Can you work these out from the drawing? Everything is in mm from the part's minimum corner. A direction names the side the tool comes from. Round coordinates to 2 decimals unless told otherwise and drop trailing zeros. Write each loop counter-clockwise with the first axis right and the second up, starting at its lowest first coordinate (ties: lowest second). Pieces come first, ordered by that corner, then holes. Notation, with made-up numbers: (81, -32.5) - (114, -32.5) arc R24 ccw to (114, -15.5) - close; hole circle Ø4 at (79, -20.5). An arc over 180 degrees is marked (long way). One line per item, written item: value. Start each with the question number.
Item 1: Thinking about a two-plate mould opening in Y: for the marked faces 1, 2 and 3, which applies, released by +Y, released by -Y, zero draft, split by the parting line, or undercut?
Item 2: For the marked faces 4, 5 and 6, which set-ups out of +Z, -Z, +X, -X, +Y, -Y let a thin tool reach every point of the face, with its end or its side?
Item 3: Imagine slicing it at B-B, the plane z = 1.5. Please give me the cut outline in (x, y), then the cut area to 3 significant figures.
Item 4: If I drill on line 1 (Z direction, x = 2.5, y = 20) (3 decimals); line 2 (Z direction, x = 2.5, y = 43) (3 decimals); line 3 (Y direction, x = 4, z = 5.75), over which ranges is the centre line in solid material (lowest first)?
Item 5: Imagine slicing it at A-A, the plane x = 10.5. Please give me the cut outline in (y, z) (3 decimals).
Item 6: Imagine slicing it at C-C, the plane y = 52.5. Please give me the cut outline in (x, z).
Item 7: For P1, Ø3, axis at x = 20.5, y = 66.5, coming from the -Z side (3 decimals), with a flat end and sliding along its axis, tell me the tip position at first contact or that it passes through.
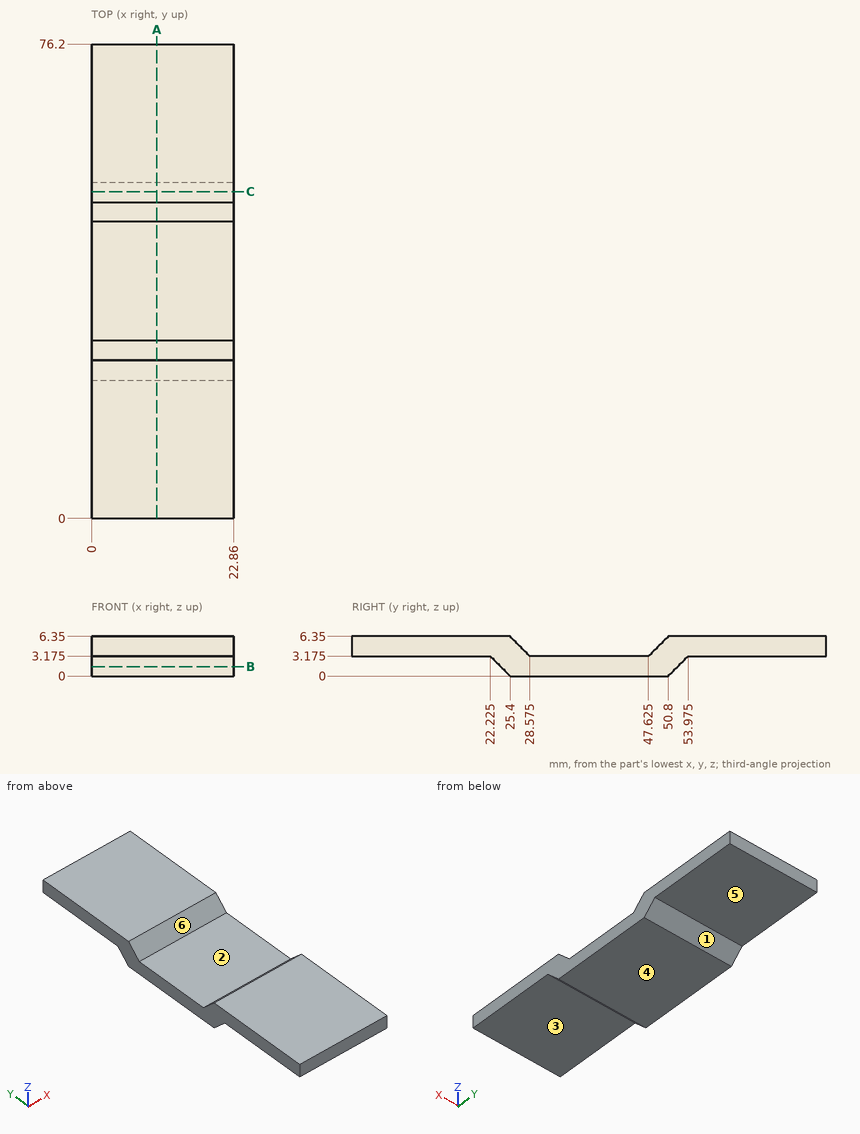
Values follow:
1. face 1: released by +Y
1. face 2: undercut
1. face 3: zero draft
2. face 4: -Z, +X, -X, +Y, -Y
2. face 5: -Z, +X, -X, +Y
2. face 6: +Z, +X, -X
3. outline: (0, 23.9) - (22.86, 23.9) - (22.86, 52.3) - (0, 52.3) - close
3. area: 649 mm^2
4. line 1: z = 3.175 to 6.35
4. line 2: z = 0 to 3.175
4. line 3: y = 0 to 26, 50.2 to 76.2
5. outline: (0, 3.175) - (22.225, 3.175) - (25.4, 0) - (50.8, 0) - (53.975, 3.175) - (76.2, 3.175) - (76.2, 6.35) - (50.8, 6.35) - (47.625, 3.175) - (28.575, 3.175) - (25.4, 6.35) - (0, 6.35) - close
6. outline: (0, 1.7) - (22.86, 1.7) - (22.86, 6.35) - (0, 6.35) - close
7. P1: stops at z = 3.175
